Design review of the part built by this model. Coordinates are the model's own, in mm. A direction names the side the tool comes from. Coordinates: 2 decimals unless noted, no trailing zeros. Loops run counter-clockwise (first coordinate to the right, second up) from the corner with the lowest first, then second, coordinate; pieces in that order, holes last.
Q1. Add section B-B on x = 192.5. Give the boundary of the cut face in (y, z).
Q2. Draft analysis for pull direction Z (two halves, no side actions). For faces 1 (the face through (7, -15, 175)), 2 (the face through (-142, -288, -175)), 3 (the face through (218, -288, 2)), 4 (the face through (-428, -144, 2)), state which applies: released by +Z, released by -Z, zero draft, split by the parting line, or undercut.
Q3. Add section A-A on z = -49. Give the boundary of the cut face in (x, y), and give its area (3 significant figures).
Q4. For P1, Ø3, axis at y = -240, z = -28, coming from the +X side; P2, Ø12, axis at y = -240, z = -8.5, coming from the +X side; P3, Ø12, axis at x = 138, y = -74.5, coming from the +Z side, all flat-tipped, find the tip position at first contact; note any pin that passes through.
Q5. Machinability: for faces 5 (the face through (-192, -275, 130)), 6 (the face through (-438, -154, -2)), 7 (the face through (438, -43, 2)), 8 (the face through (428, -26, -2)), 9 (the face through (-6, -154, 120)), which of the approach directions +Z, -Z, +X, -X, +Y, -Y give a long, thin tool a straight path to every point of the face, cutting with its end or side? Answer none if there is none.
Q6. Wall thickness on probe 1 along Z at (x, y) = (142, -20); probe 2 along Z at (x, y) = (-220.5, -181); probe 3 along X at (y, z) = (-35, -52.5): over which ranges is each line inside the solid? List them lowest first.
Q7. Add section C-C on y = -179. Give the boundary of the cut face in (x, z), and give its area (3 significant figures).
Q8. Add section D-D on y = -121. Give the boundary of the cut face in (x, z).
Autodesk Inventor part; units mm, degrees
ref_plane "YZ Plane" through (0, 0, 0) normal (1, 0, 0) x (0, 1, 0)
ref_plane "XZ Plane" through (0, 0, 0) normal (0, 1, 0) x (-1, 0, 0)
ref_plane "XY Plane" through (0, 0, 0) normal (0, 0, 1) x (1, 0, 0)
sketch "Эскиз1" plane through (0, 0, 0) normal (0, 1, 0) x (-1, 0, 0)
  line L0 (493, -175) -> (-493, -175)
  line L1 (-493, -175) -> (-493, 175)
  line L2 (-493, 175) -> (493, 175)
  line L3 (493, 175) -> (493, -175)
  line L4 (493, -175) -> (-493, 175) construction
  line L5 (-493, -175) -> (493, 175) construction
  point P0 (0, 0)
  dimension "d0" = 986
  dimension "d1" = 350
extrude "Выдавливание1" add sketch "Эскиз1" against normal blind 300
sketch "Эскиз2" plane through (0, -300, 0) normal (0, -1, 0) x (1, 0, 0)
  line L0 (493, 175) -> (-493, 175)
  line L1 (-493, 175) -> (-493, -175)
  line L2 (-493, -175) -> (493, -175)
  line L3 (493, -175) -> (493, 175)
  line L4 (-438, 120) -> (438, 120)
  line L5 (438, 120) -> (438, -120)
  line L6 (438, -120) -> (-438, -120)
  line L7 (-438, -120) -> (-438, 120)
  point P0 (0, 0)
  dimension "d4" = 55
extrude "Выдавливание2" cut sketch "Эскиз2" against normal blind 270
sketch "Эскиз4" plane through (-493, 0, 175) normal (0, 0, 1) x (1, 0, 0)
  line L0 (0, 0) -> (986, 0)
  line L1 (986, 0) -> (711, -275)
  line L2 (986, 0) -> (1374.9087, 0) construction
  line L3 (931, -300) -> (55, -300)
  line L4 (931, -55) -> (931, -300)
  line L5 (931, -300) -> (931, -30)
  line L6 (711, -275) -> (711, -300)
  line L7 (711, -300) -> (931, -300)
  point P0 (493, 0)
  dimension "d10" = 135
  dimension "d13" = 25
extrude "Выдавливание3" cut sketch "Эскиз4" against normal through all
sketch "Эскиз5" plane through (0, -300, 0) normal (0, -1, 0) x (1, 0, 0)
  line L0 (-493, -175) -> (-493, 175) construction
  line L1 (493, -175) -> (-493, -175) construction
  line L2 (493, 175) -> (493, -175) construction
  line L3 (-493, 175) -> (493, 175) construction
  line L4 (438, 120) -> (-438, 120) construction
  line L5 (438, -120) -> (438, 120) construction
  line L6 (-438, -120) -> (438, -120) construction
  line L7 (-438, 120) -> (-438, -120) construction
  line L8 (-493, 175) -> (493, 175)
  line L9 (218, 175) -> (-493, 175)
  line L10 (-493, -175) -> (-493, 175)
  line L11 (-493, 175) -> (-493, -175)
  line L12 (-493, -175) -> (218, -175)
  line L13 (493, -175) -> (-493, -175)
  line L14 (218, 175) -> (218, -175)
  point P0 (0, 0)
  point P1 (218, 120)
extrude "Выдавливание5" add sketch "Эскиз5" against normal blind 25
shell "Оболочка1" thickness 10 removed faces 1 at (-164.3333, 0, -58.3333)
sketch "Эскиз6" plane through (-483, -20, 165) normal (0, 1, 0) x (1, 0, 0)
  line L0 (0, 330) -> (0, 0)
  line L1 (0, 0) -> (966, 0)
  line L2 (966, 0) -> (966, 330)
  line L3 (966, 330) -> (0, 330)
  line L4 (911, 55) -> (55, 55)
  line L5 (55, 55) -> (55, 275)
  line L6 (55, 275) -> (911, 275)
  line L7 (911, 275) -> (911, 55)
  point P0 (483, 165)
extrude "Выдавливание6" add sketch "Эскиз6" along normal up to surface (20 mm away)
sketch "Эскиз7" plane through (-483, -290, -165) normal (0, 1, 0) x (1, 0, 0)
  line L0 (691, 0) -> (691, -330)
  line L1 (0, 0) -> (691, 0)
  line L2 (0, -330) -> (0, 0)
  line L3 (691, -330) -> (0, -330)
  point P0 (483, -165)
extrude "Выдавливание7" add sketch "Эскиз7" along normal up to surface (5 mm away)
sketch "Эскиз8" plane through (-493, 0, 175) normal (0, 0, 1) x (1, 0, 0)
  line L0 (0, 0) -> (986, 0)
  line L1 (986, 0) -> (986, -30)
  point P0 (493, 0)
  point P1 (856, 0)
  point P2 (656, 0)
  point P3 (356, 0)
  point P4 (986, -15)
  dimension "d21" = 130
  dimension "d22" = 200
  dimension "d23" = 300
properties part number "Корпус" material "Сталь, углеродистая"
Entries:
1. outline: (-300, -175) - (-275, -175) - (-275, -120) - (-30, -120) - (-30, -175) - (0, -175) - (0, -110) - (-285, -110) - (-285, 110) - (0, 110) - (0, 175) - (-30, 175) - (-30, 120) - (-275, 120) - (-275, 175) - (-300, 175) - close
2. face 1: released by +Z
2. face 2: released by -Z
2. face 3: zero draft
2. face 4: undercut
3. outline: (-493, -300) - (218, -300) - (218, -275) - (438, -55) - (438, -30) - (493, -30) - (493, 0) - (428, 0) - (428, -50.86) - (208, -270.86) - (208, -285) - (-428, -285) - (-428, 0) - (-493, 0) - (-493, -30) - (-438, -30) - (-438, -275) - (-493, -275) - close
3. area: 21,100 mm2
4. P1: stops at x = 254.5
4. P2: stops at x = 259
4. P3: stops at z = 120
5. face 5: -X
5. face 6: +Z, -Z, -X
5. face 7: +Z, -Z, +X, -Y
5. face 8: +Y
5. face 9: +Z, +X, -X
6. probe 1: z = -175 to -110, 110 to 175
6. probe 2: z = -120 to -110, 110 to 120
6. probe 3: x = -438 to -428, 428 to 438
7. outline: (-438, -120) - (314, -120) - (314, 120) - (-438, 120) - close; hole (-428, -110) - (299.86, -110) - (299.86, 110) - (-428, 110) - close
7. area: 20,400 mm2
8. outline: (-438, -120) - (372, -120) - (372, 120) - (-438, 120) - close; hole (-428, -110) - (357.86, -110) - (357.86, 110) - (-428, 110) - close
